```python
from build123d import *

# Parameters (mm, degrees)
BOSS_EXTRUDE1_DEPTH         = 30
SKETCH2_R                   = 4
CUT_EXTRUDE1_DEPTH          = 31
SKETCH3_R                   = 7
CUT_EXTRUDE2_DEPTH          = 1
SKETCH4_R                   = 7
CUT_EXTRUDE3_DEPTH          = 1
TAP_DRILL_FOR_M4X0_7_TAP1_D = 3.3


with BuildPart() as part:
    # Sketch1 → Boss-Extrude1 (new body)
    with BuildSketch(Plane.XY):
        Polygon((-17, -2.405243596), (-17, -8.405243596), (-7, -8.405243596), (-6.5, -7.905243596), (6.5, -7.905243596), (7, -8.405243596), (17, -8.405243596), (17, -2.405243596), (16, -1.405243596), (16, 8.594756404), (15, 9.594756404), (7.5, 9.594756404), (4.5, 13.594756404), (-4.5, 13.594756404), (-7.5, 9.594756404), (-15, 9.594756404), (-16, 8.594756404), (-16, -1.405243596), align=None)
    extrude(amount=BOSS_EXTRUDE1_DEPTH)

    # Sketch2 → Cut-Extrude1 (cut, through all)
    with BuildSketch(Plane(origin=(0, 0, 0), x_dir=(-1, 0, 0), z_dir=(0, 0, -1))):
        with Locations((0, 2.594756404)):
            Circle(SKETCH2_R)
    extrude(amount=-CUT_EXTRUDE1_DEPTH, mode=Mode.SUBTRACT)

    # Sketch3 → Cut-Extrude2 (cut)
    with BuildSketch(Plane(origin=(0, 0, 0), x_dir=(-1, 0, 0), z_dir=(0, 0, -1))):
        with Locations((0, 2.594756404)):
            Circle(SKETCH3_R)
    extrude(amount=-CUT_EXTRUDE2_DEPTH, mode=Mode.SUBTRACT)

    # Sketch4 → Cut-Extrude3 (cut)
    with BuildSketch(Plane.XY.offset(30)):
        with Locations((0, 2.594756404)):
            Circle(SKETCH4_R)
    extrude(amount=-CUT_EXTRUDE3_DEPTH, mode=Mode.SUBTRACT)

    # Tap Drill for M4x0.7 Tap1 (through all)
    with Locations(Plane(origin=(0, -8.405243596, 0), x_dir=(-1, 0, 0), z_dir=(0, -1, 0))):
        with Locations((-12, -6), (12, -6), (12, -24), (-12, -24)):
            Hole(TAP_DRILL_FOR_M4X0_7_TAP1_D / 2)


solid = part.part
```
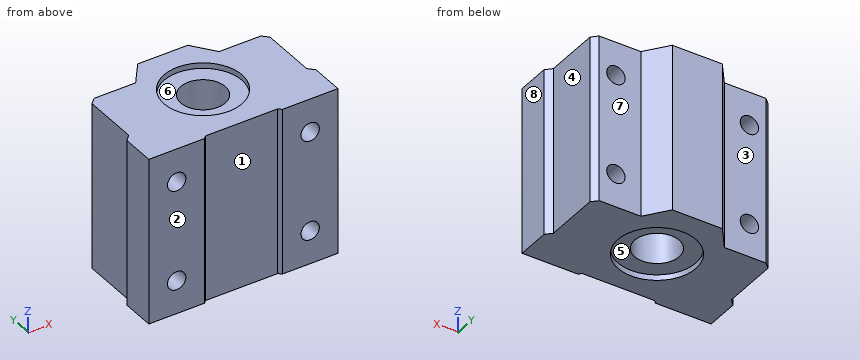
Check sheet for the modelled part. Datum: model origin and axes. Units: mm. Face numbers are marked on the shaded views. A direction names the side the tool comes from. Give positions to 0.01 mm unless a question says otherwise; leave off trailing zeros. Order: outer loops, then holes, each group sorted by start corner. A loop starts at its lowest first (then second) coordinate and runs counter-clockwise, first axis right, second up. Notation, with made-up numbers: (-27.75, 64) -> (31.25, 64) arc R11 ccw to (31.25, 75) -> close; hole circle Ø11 at (7, 54.5). An arc over 180 degrees is marked (long way). Use CSV: the item, a comma, the result in double quotes. Start each with the question number.
1) Sectioned sample at C-C, the plane y = -5.75. Record the boundary of the cut face in (x, z), plus the area to 3 significant figures.
2) Mould release check, pull along Y, two halves, no side actions. Record for the marked faces 6, 7 and 8: released by +Y, released by -Y, zero draft, split by the parting line, or undercut.
3) Sectioned sample at A-A, the plane z = 24. Record the boundary of the cut face in (x, y).
4) Set-up check for the marked faces 1, 2, 3, 4 and 5: record each of +Z, -Z, +X, -X, +Y, -Y from which the full face is reachable in a straight line by a thin tool's end or side.
5) Sectioned sample at D-D, the plane x = 12. Record the boundary of the cut face in (y, z).
6) Sectioned sample at B-B, the plane x = 0. Record the boundary of the cut face in (y, z), plus the area to 3 significant figures.
7) Material ranges on line 1 (Z direction, x = -12, y = 0.75); line 2 (X direction, y = -3.75, z = 24); line 3 (Z direction, x = 13, y = 9.5), recorded low to high. Write a range as from..to.
8) Go/stop test with flat-tipped pins: P1, Ø5, axis at x = 5.5, z = 16.5, coming from the -Y side; P2, Ø3, axis at y = 1, z = 9.5, coming from the -X side; P3, Ø6.5, axis at x = -3, z = 11, coming from the -Y side; P4, Ø3, axis at y = 11.5, z = 9, coming from the -X side. Record where each tip stops, or that it passes through.
Recorded:
1,outline,"(-17, 0) -> (17, 0) -> (17, 30) -> (-17, 30) -> close; hole circle Ø3.3 at (-12, 6); hole circle Ø3.3 at (-12, 24); hole circle Ø3.3 at (12, 6); hole circle Ø3.3 at (12, 24)"
1,area,"986 mm2"
2,face 6,"undercut"
2,face 7,"released by +Y"
2,face 8,"zero draft"
3,outline,"(-17, -8.41) -> (-13.65, -8.41) -> (-13.65, 9.59) -> (-15, 9.59) -> (-16, 8.59) -> (-16, -1.41) -> (-17, -2.41) -> close; (-10.35, -8.41) -> (-7, -8.41) -> (-6.5, -7.91) -> (6.5, -7.91) -> (7, -8.41) -> (10.35, -8.41) -> (10.35, 9.59) -> (7.5, 9.59) -> (4.5, 13.59) -> (-4.5, 13.59) -> (-7.5, 9.59) -> (-10.35, 9.59) -> close; (13.65, -8.41) -> (17, -8.41) -> (17, -2.41) -> (16, -1.41) -> (16, 8.59) -> (15, 9.59) -> (13.65, 9.59) -> close; hole circle Ø8 at (0, 2.59)"
4,face 1,"+Z, -Z, -Y"
4,face 2,"+Z, -Z, +X, -X, -Y"
4,face 3,"+Z, -Z, -X, +Y"
4,face 4,"+Z, -Z, +X, +Y"
4,face 5,"-Z"
5,outline,"(-8.41, 0) -> (9.59, 0) -> (9.59, 4.35) -> (-8.41, 4.35) -> close; (-8.41, 7.65) -> (9.59, 7.65) -> (9.59, 22.35) -> (-8.41, 22.35) -> close; (-8.41, 25.65) -> (9.59, 25.65) -> (9.59, 30) -> (-8.41, 30) -> close"
6,outline,"(-7.91, 0) -> (-4.41, 0) -> (-4.41, 1) -> (-1.41, 1) -> (-1.41, 29) -> (-4.41, 29) -> (-4.41, 30) -> (-7.91, 30) -> close; (6.59, 1) -> (9.59, 1) -> (9.59, 0) -> (13.59, 0) -> (13.59, 30) -> (9.59, 30) -> (9.59, 29) -> (6.59, 29) -> close"
6,area,"393 mm2"
7,line 1,"0..4.35, 7.65..22.35, 25.65..30"
7,line 2,"-17..-13.65, -10.35..10.35, 13.65..17"
7,line 3,"0..4.69, 7.31..22.69, 25.31..30"
8,P1,"y = -8.41"
8,P2,"x = -16"
8,P3,"y = -7.91"
8,P4,"x = -7.2"
